Read the model definition and answer for the solid it produces. Units are mm, in the model's axes. Face numbers are marked on the shaded views. A direction names the side the tool comes from. Coordinates: 2 decimals unless noted, no trailing zeros. Order: outer loops, then holes, each group sorted by start corner. A loop starts at its lowest first (then second) coordinate and runs counter-clockwise, first axis right, second up. Notation, with made-up numbers: (0.5, 1) -> (57.5, 1) arc R30 cw to (57.5, 25) -> close; hole circle Ø6 at (-5.5, -24.5). An arc over 180 degrees is marked (long way). Return JSON: item names as keys, results as strings. Group by question number.
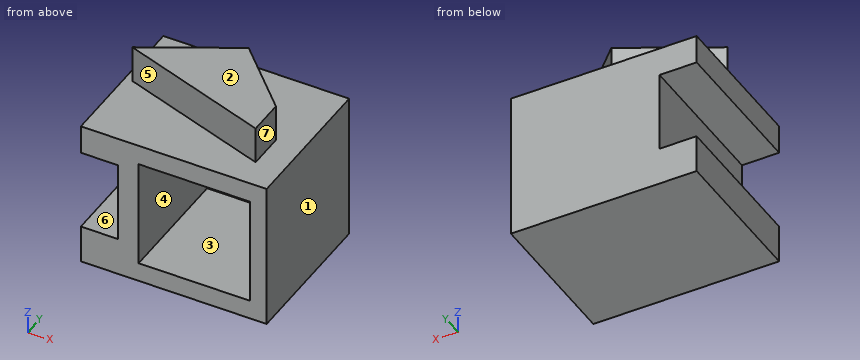
```python
from build123d import *

# Parameters (mm, degrees)
F0_W     = 100
F0_H     = 100
F1_DEPTH = 100
F2_W     = 75.0674530864
F2_H     = 73.3678080142
F3_DEPTH = 83
F4_W     = 100
F4_H     = 25.7778791711
F5_DEPTH = 25
F6_W     = 100
F6_H     = 19.5503592491
F7_DEPTH = 25
F9_DEPTH = 25


# Not quite as in the source:
# - the program builds the solid bodies; features that only make, move or delete a surface that nothing else refers to are left out


with BuildPart() as f1:
    # F0 (on Front) → F1 (new body)
    with BuildSketch(Plane.XZ):
        with Locations((17.8484685719, 11.3331817091)):
            Rectangle(F0_W, F0_H)
    extrude(amount=F1_DEPTH)

    # F2 (on face) → F3 (cut)
    with BuildSketch(Plane.XZ.offset(100)):
        with Locations((19.2625932395, 11.0476631671)):
            Rectangle(F2_W, F2_H)
    extrude(amount=-F3_DEPTH, mode=Mode.SUBTRACT)

    # F4 (on face) → F5 (join)
    with BuildSketch(Plane(origin=(-32.1515314281, 0, 0), x_dir=(0, -1, 0), z_dir=(-1, 0, 0))):
        with Locations((50, -25.7778787054)):
            Rectangle(F4_W, F4_H)
    extrude(amount=F5_DEPTH)

    # F6 (on face) → F7 (join)
    with BuildSketch(Plane(origin=(-32.1515314281, 0, 0), x_dir=(0, -1, 0), z_dir=(-1, 0, 0))):
        with Locations((50, 51.5580020845)):
            Rectangle(F6_W, F6_H)
    extrude(amount=F7_DEPTH)

    # F8 (on face) → F9 (join)
    with BuildSketch(Plane.XY.offset(61.3331817091)):
        Polygon((8.1979809329, -14.2997056246), (-51.9804432988, -46.9225756824), (49.6200919151, -80.5339738727), (49.6200919151, -55.9161007404), align=None)
    extrude(amount=F9_DEPTH)


solid = f1.part
```
1. Find section C-C on y = -38.5. Determine the outline of the cut face in (x, z), and give its area (3 significant figures).
2. For a pull along Z with two mould halves and no side action, classify the marked faces 1, 2, 3 and 4 as released by +Z, released by -Z, zero draft, split by the parting line, or undercut.
3. Find section D-D on x = 24. Determine the outline of the cut face in (y, z), and give its area (3 significant figures).
4. Find section A-A on y = -10.5. Determine the outline of the cut face in (x, z).
5. Straight lines are drawn through the part: L1, parallel to X at y = -63, z = 12; L2, parallel to Z at x = -44, y = -34; L3, parallel to X at y = -82, z = -16.5. For each, find the intervals that lie inside material, in ascending order.
6. Find section B-B on z = -2. Determine the outline of the cut face in (x, y), and give its area (3 significant figures).
7. Given pin 1 (6 mm diameter, centred on x = -6, z = 44.5, fed in from -Y); pin 2 (12.5 mm diameter, centred on y = -72, z = 72.5, fed in from +X), each flat-ended and moving along its own axis, determine where each tip first touches the part or whether it passes through.
8. Which of the six approach directions +Z, -Z, +X, -X, +Y, -Y give full straight-line access (tool end or side, diameter ignored) to the marked faces 5, 6 and 7?
Result:
{
 "1": {"outline": "(-57.15, -38.67) -> (67.85, -38.67) -> (67.85, 61.33) -> (32.29, 61.33) -> (32.29, 86.33) -> (-36.44, 86.33) -> (-36.44, 61.33) -> (-57.15, 61.33) -> (-57.15, 41.78) -> (-32.15, 41.78) -> (-32.15, -12.89) -> (-57.15, -12.89) -> close; hole (-18.27, -25.64) -> (56.8, -25.64) -> (56.8, 47.73) -> (-18.27, 47.73) -> close", "area": "7,340 mm^2"},
 "2": {"face 1": "zero draft", "face 2": "released by +Z", "face 3": "undercut", "face 4": "undercut"},
 "3": {"outline": "(-100, -38.67) -> (0, -38.67) -> (0, 61.33) -> (-30.18, 61.33) -> (-30.18, 86.33) -> (-72.06, 86.33) -> (-72.06, 61.33) -> (-100, 61.33) -> (-100, 47.73) -> (-17, 47.73) -> (-17, -25.64) -> (-100, -25.64) -> close", "area": "4,960 mm^2"},
 "4": {"outline": "(-57.15, -38.67) -> (67.85, -38.67) -> (67.85, 61.33) -> (-57.15, 61.33) -> (-57.15, 41.78) -> (-32.15, 41.78) -> (-32.15, -12.89) -> (-57.15, -12.89) -> close"},
 "5": {"L1": "-32.15 to -18.27, 56.8 to 67.85", "L2": "-38.67 to -12.89, 41.78 to 61.33", "L3": "-57.15 to -18.27, 56.8 to 67.85"},
 "6": {"outline": "(-32.15, -100) -> (-18.27, -100) -> (-18.27, -17) -> (56.8, -17) -> (56.8, -100) -> (67.85, -100) -> (67.85, 0) -> (-32.15, 0) -> close", "area": "3,770 mm^2"},
 "7": {"pin 1": "y = -17", "pin 2": "x = 49.62"},
 "8": {"face 5": "+Z, -X, -Y", "face 6": "-X, +Y, -Y", "face 7": "+Z, +X, +Y, -Y"}
}
